The listing builds one solid part. Answer for the finished solid, in the listing's coordinates (mm). Face numbers are marked on the shaded views. A direction names the side the tool comes from. Give positions to 0.01 mm unless a question says otherwise; leave off trailing zeros. Loops run counter-clockwise (first coordinate to the right, second up) from the corner with the lowest first, then second, coordinate; pieces in that order, holes last. Notation, with made-up numbers: M 30.25,63 L 74.25,63 A3 ccw 74.25,67 Z; hole C 67.25,29.5 d4. An arc over 180 degrees is marked long. One line per item, written item: value. Start each with the question number.
Q1. A cutting plane is placed at A-A, the plane y = 0. Determine the outline of the cut face in (x, z).
Q2. Flat-ended cylindrical pins translate along their axes: pin 1 (7 mm diameter, centred on x = 23.5, y = -21, fed in from +Z); pin 2 (6.5 mm diameter, centred on x = 42, z = 10, fed in from +Y); pin 3 (4 mm diameter, centred on y = -42.5, z = 18, fed in from +X). Find the tip coordinate at first contact, or state that the pin passes through.
Q3. A cutting plane is placed at C-C, the plane z = 18.75. Determine the outline of the cut face in (x, y), and give its area (3 significant figures).
Q4. The mould has two halves that part along Y. Classify the marked faces 5, 6 and 7: +Y half, -Y half, draft (parallel to the pull), parting line (faces both ways), or undercut.
Q5. Consider L1, parallel to Y at x = 8, z = 3.75; L2, parallel to X at y = -43, z = 3; L3, parallel to Y at x = 2.5, z = 1.5. Determine where each line is inside the solid, lowest interval first.
Q6. A cutting plane is placed at D-D, the plane y = -8.5. Determine the outline of the cut face in (x, z).
Q7. For the marked faces 1, 2, 3 and 4, determine the directions among +Z, -Z, +X, -X, +Y, -Y from which every point of the face is accessible in a straight line to the end or side of a thin tool.
Q8. A cutting plane is placed at B-B, the plane x = 25. Determine the outline of the cut face in (y, z).
from build123d import *

# Parameters (mm, degrees)
SKETCH1_W           = 33
SKETCH1_H           = 66
BOSS_EXTRUDE1_DEPTH = 8
SKETCH3_R           = 2.75
SKETCH3_R_2         = 11.6
CUT_EXTRUDE1_DEPTH  = 62.269894728
BOSS_EXTRUDE3_START = 2.5
SKETCH4_R           = 4.25
SKETCH4_R_2         = 2.75
BOSS_EXTRUDE3_DEPTH = 2.5
SKETCH6_R           = 12.1
CUT_EXTRUDE2_DEPTH  = 5.1
CUT_EXTRUDE6_DEPTH  = 62.646167764
SKETCH10_R          = 2.75
BOSS_EXTRUDE4_DEPTH = 7
CUT_EXTRUDE3_DEPTH  = 6
SKETCH12_R          = 2.75
CUT_EXTRUDE4_DEPTH  = 6
FILLET7_R           = 2
FILLET5_R           = 25
FILLET6_R           = 5.8
SKETCH15_R          = 3.5
SKETCH15_R_2        = 2.25
BOSS_EXTRUDE5_DEPTH = 8
CUT_EXTRUDE5_DEPTH  = 5
FILLET8_R           = 2


with BuildPart() as part:
    # Sketch1 → Boss-Extrude1 (new body)
    with BuildSketch(Plane.XY):
        with Locations((16.5, -18)):
            Rectangle(SKETCH1_W, SKETCH1_H)
    extrude(amount=BOSS_EXTRUDE1_DEPTH)

    # Sketch3 → Cut-Extrude1 (cut, through all)
    with BuildSketch(Plane.XY.offset(8)):
        with Locations((25, -20)):
            Circle(SKETCH3_R)
        Circle(SKETCH3_R_2)
        with BuildLine():
            Line((-17.5, 0), (-32.5, 0))
            ThreePointArc((-32.5, 0), (-18.056032573, -27.0227624), (12.437211552, -30.026084807))
            ThreePointArc((12.437211552, -30.026084807), (16.496182303, -20.22686257), (6.696960066, -16.167891819))
            ThreePointArc((6.696960066, -16.167891819), (-9.722479078, -14.550718215), (-17.5, 0))
        make_face()
    extrude(amount=-CUT_EXTRUDE1_DEPTH, mode=Mode.SUBTRACT)

    # Sketch4 → Boss-Extrude3 (add)
    with BuildSketch(Plane.XY.offset(8).offset(BOSS_EXTRUDE3_START)):
        with Locations((25, -20)):
            Circle(SKETCH4_R)
        with Locations((25, -20)):
            Circle(SKETCH4_R_2, mode=Mode.SUBTRACT)
    extrude(amount=-BOSS_EXTRUDE3_DEPTH)

    # Sketch6 → Cut-Extrude2 (cut)
    with BuildSketch(Plane(origin=(0, 0, 0), x_dir=(-1, 0, 0), z_dir=(0, 0, -1))):
        Circle(SKETCH6_R)
    extrude(amount=-CUT_EXTRUDE2_DEPTH, mode=Mode.SUBTRACT)

    # Sketch17 → Cut-Extrude6 (cut, through all)
    with BuildSketch(Plane(origin=(0, 0, 0), x_dir=(-1, 0, 0), z_dir=(0, 0, -1))):
        with BuildLine():
            Line((0, 15), (0, 35))
            Line((0, 35), (-33, 35))
            Line((-33, 35), (-33, -3))
            ThreePointArc((-33, -3), (-29.485281374, 5.485281374), (-21, 9))
            ThreePointArc((-21, 9), (-14.200652085, 9.952282296), (-7.924528302, 12.735849057))
            ThreePointArc((-7.924528302, 12.735849057), (-4.120816918, 14.422859215), (0, 15))
        make_face()
    extrude(amount=-CUT_EXTRUDE6_DEPTH, mode=Mode.SUBTRACT)

    # Sketch10 → Boss-Extrude4 (add)
    with BuildSketch(Plane.XZ.offset(51)):
        with BuildLine():
            Line((42, 0), (32, 0))
            Line((32, 0), (32, 10))
            ThreePointArc((32, 10), (49.071067812, 17.071067812), (42, 0))
        make_face()
        with Locations(Location((42, 10, 0), (0, 0, 270))):
            Circle(SKETCH10_R, mode=Mode.SUBTRACT)
    extrude(amount=-BOSS_EXTRUDE4_DEPTH)

    # Sketch11 → Cut-Extrude3 (cut)
    with BuildSketch(Plane.XY.offset(8)):
        with BuildLine():
            Line((0, -51), (24, -51))
            Line((24, -51), (24, -43))
            ThreePointArc((24, -43), (21.656854249, -37.343145751), (16, -35))
            Line((16, -35), (0, -35))
            Line((0, -35), (0, -51))
        make_face()
    extrude(amount=-CUT_EXTRUDE3_DEPTH, mode=Mode.SUBTRACT)

    # Sketch12 → Cut-Extrude4 (cut)
    with BuildSketch(Plane.XY.offset(2)):
        with Locations((8, -43)):
            Circle(SKETCH12_R)
    extrude(amount=-CUT_EXTRUDE4_DEPTH, mode=Mode.SUBTRACT)

    # Fillet7
    fillet7_edges = [part.edges().sort_by_distance(p)[0] for p in [
        (8, -35, 2),
        (21.656854249, -37.343145751, 2),
        (24, -47, 2),
    ]]
    fillet(fillet7_edges, radius=FILLET7_R)

    # Fillet5
    # the kernel refuses this fillet: 25 mm, written as the material it adds along each edge
    with BuildSketch(Plane(origin=(32, -44, 8), x_dir=(-1, 0, 0), z_dir=(0, -1, 0))) as fillet5_piece_1:
        with BuildLine():
            CenterArc((18.096713956, -22.870425604), FILLET5_R, 113.820244592, 29.574545381)
            Line((-1.972367441, -7.962978744), (-3.979275581, -6.472234058))
            ThreePointArc((-3.979275581, -6.472234058), (-2.5, -2), (-2.5, 0))
            Line((-2.5, 0), (0, 2.5))
            ThreePointArc((0, 2.5), (4, 2.5), (6.990328604, 2.28704256))
            Line((6.990328604, 2.28704256), (8, 0))
        make_face()
    extrude(amount=7)

    # Fillet6
    # the kernel refuses this fillet: 5.8 mm, written as the material it adds along each edge
    with BuildSketch(Plane(origin=(33, -44, 0), x_dir=(0, 1, 0), z_dir=(0, 0, 1))) as fillet6_piece_1:
        with BuildLine():
            CenterArc((FILLET6_R, -FILLET6_R), FILLET6_R, 90, 90)
            Line((0, -FILLET6_R), (0, 0))
            Line((0, 0), (FILLET6_R, 0))
        make_face()
    extrude(amount=8)
    with BuildSketch(Plane(origin=(33, -44, 8), x_dir=(0, 1, 0), z_dir=(-1, 0, 0))) as fillet6_piece_2_section:
        with BuildLine():
            CenterArc((FILLET6_R, -FILLET6_R), FILLET6_R, 90, 90)
            Line((0, -FILLET6_R), (0, 0))
            Line((0, 0), (FILLET6_R, 0))
        make_face()
    fillet6_piece_2 = extrude(amount=23.5, mode=Mode.PRIVATE)
    fillet6_piece_2 = fillet6_piece_2 - Plane(origin=(13.903286044, -44, 30.870425604), x_dir=(-1, 0, 0), z_dir=(0, 1, 0)) * Cylinder(25, 71, mode=Mode.PRIVATE)
    add(fillet6_piece_2)
    with BuildSketch(Plane(origin=(47.5, -44, 8), x_dir=(0, 1, 0), z_dir=(-1, 0, 0))) as fillet6_piece_3a_section:
        with BuildLine():
            CenterArc((FILLET6_R, -FILLET6_R), FILLET6_R, 90, 90)
            Line((0, -FILLET6_R), (0, 0))
            Line((0, 0), (FILLET6_R, 0))
        make_face()
    fillet6_piece_3a = extrude(amount=23.5, mode=Mode.PRIVATE)
    fillet6_piece_3a = fillet6_piece_3a - Plane(origin=(42, -44, 10), x_dir=(0, 0, -1), z_dir=(0, -1, 0)) * Cylinder(2.75, 71, mode=Mode.PRIVATE)
    fillet6_piece_3a = split(fillet6_piece_3a, bisect_by=Plane(origin=(33, -44, 8), z_dir=(1, 0, 0)), keep=Keep.TOP, mode=Mode.PRIVATE)
    with BuildSketch(Plane(origin=(33, -44, 0), x_dir=(0, 1, 0), z_dir=(0, 0, 1))) as fillet6_piece_3b_section:
        with BuildLine():
            CenterArc((FILLET6_R, -FILLET6_R), FILLET6_R, 90, 90)
            Line((0, -FILLET6_R), (0, 0))
            Line((0, 0), (FILLET6_R, 0))
        make_face()
    fillet6_piece_3b = extrude(amount=22.5, mode=Mode.PRIVATE)
    fillet6_piece_3b = split(fillet6_piece_3b, bisect_by=Plane(origin=(33, -44, 8), z_dir=(0, 0, 1)), keep=Keep.TOP, mode=Mode.PRIVATE)
    fillet6_piece_3b = fillet6_piece_3b & Plane(origin=(42, -44, 10), x_dir=(-1, 0, 0), z_dir=(0, -1, 0)) * Cylinder(10, 69, mode=Mode.PRIVATE)
    fillet6_piece_3 = fillet6_piece_3a & fillet6_piece_3b
    add(fillet6_piece_3)

    # Sketch15 → Boss-Extrude5 (add)
    with BuildSketch(Plane.XY):
        with Locations(Location((8, -43, 0), (0, 0, 180))):
            Circle(SKETCH15_R)
        with Locations(Location((8, -43, 0), (0, 0, 180))):
            Circle(SKETCH15_R_2, mode=Mode.SUBTRACT)
    extrude(amount=BOSS_EXTRUDE5_DEPTH)

    # Sketch13 → Cut-Extrude5 (cut)
    with BuildSketch(Plane(origin=(0, 0, 0), x_dir=(-1, 0, 0), z_dir=(0, 0, -1))):
        Polygon((-22.546261356, -15.75), (-27.453738644, -15.75), (-29.907477288, -20), (-27.453738644, -24.25), (-22.546261356, -24.25), (-20.092522712, -20), align=None)
    extrude(amount=-CUT_EXTRUDE5_DEPTH, mode=Mode.SUBTRACT)

    # Fillet8
    fillet8_edges = [part.edges().sort_by_distance(p)[0] for p in [
        (11.5, -43, 2),
        (20.75, -20, 8),
    ]]
    fillet(fillet8_edges, radius=FILLET8_R)

    # Mirror1: part across plane


with BuildPart() as part_1:
    add(part.part)
    add(part.part.mirror(Plane(origin=(0, 15, 8), x_dir=(0, 0, 1), z_dir=(1, 0, 0))))


solid = part_1.part
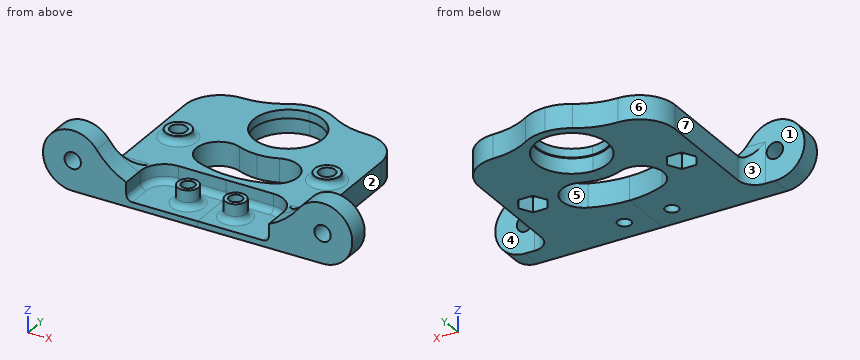
Answer block:
1. outline: M -32.62,0 L -12.1,0 L -12.1,5.1 L -11.6,5.1 L -11.6,8 L -32.62,8 Z; M 11.6,5.1 L 12.1,5.1 L 12.1,0 L 32.62,0 L 32.62,8 L 11.6,8 Z
2. pin 1: z = 10.5
2. pin 2: y = -44
2. pin 3: x = 49.44
3. outline: M -46.84,-51 L -37.16,-51 L -37.16,-44 L -46.84,-44 Z; M 37.16,-51 L 46.84,-51 L 46.84,-44 L 37.16,-44 Z
3. area: 136 mm^2
4. face 5: undercut
4. face 6: +Y half
4. face 7: draft
5. L1: -46.52 to -45.25, -40.75 to -39.48, -35.02 to -31.5, -15.76 to -9.08, 9.08 to 12.69
5. L2: -35.54 to -23.73, -11.77 to -10.25, -5.75 to -4.23, 4.23 to 5.75, 10.25 to 11.77, 23.73 to 35.54
5. L3: -51 to -32.4, -17.32 to -11.84, 11.84 to 14.79
6. outline: M -33,0 L -8.61,0 L -8.61,5.1 L -7.89,5.1 L -7.89,8 L -33,8 Z; M 7.89,5.1 L 8.61,5.1 L 8.61,0 L 33,0 L 33,8 L 7.89,8 Z
7. face 1: +Z, -X, +Y
7. face 2: +Z, -Z, +X, +Y
7. face 3: +Z, -Z, -X, +Y
7. face 4: +Z, +X, +Y
8. outline: M -51,0 L -24.25,0 L -24.25,5 L -22.75,5 L -22.75,10.5 L -24.25,10.5 L -24.25,10 A2 cw -26.25,8 L -38.2,8 A5.8 cw -40.48,8.47 L -51,8.47 Z; M -17.25,5 L -15.75,5 L -15.75,0 L 8.31,0 L 8.31,8 L -13.75,8 A2 cw -15.75,10 L -15.75,10.5 L -17.25,10.5 Z
